Read the model definition and answer for the solid it produces. Units are mm, in the model's axes. A direction names the side the tool comes from. Round coordinates to 2 decimals unless told otherwise and drop trailing zeros. Order: outer loops, then holes, each group sorted by start corner. A loop starts at its lowest first (then second) coordinate and runs counter-clockwise, first axis right, second up. Notation, with made-up numbers: (-29.75, -12.75) - (-16.75, -12.75) arc R18 ccw to (-16.75, 3.25) - close; hole circle Ø1 at (-8.75, 39.5). An arc over 180 degrees is marked (long way). Put each result on its own line as item: value. Start each with the question number.
Q1. Which of the six approach directions +Z, -Z, +X, -X, +Y, -Y give full straight-line access (tool end or side, diameter ignored) to faces 5 (the face through (-58, 2, 10.445)), 6 (the face through (32.1, 2, -57)), 7 (the face through (-10.1, 2, 22)), 8 (the face through (-32.1, 2, 58))?
Q2. For a pull along Z with two mould halves and no side action, classify faces 1 (the face through (58, 2, -50.995)), 2 (the face through (52.3, 2, -57)), 3 (the face through (58, 2, 32.445)), 4 (the face through (0.112, 1.61, 39.757)) as pulls with the +Z half, pulls with the -Z half, needs draft (parallel to the pull), parting line crosses it, or undercut.
Q3. Each of these flat-tipped pins is pushed along its axis until it touches: pin 1 Ø1.5 at (y, z) = (1, -20.5) entering from +X; pin 2 Ø1 at (y, z) = (2, -19) entering from -X; pin 3 Ø1.6 at (x, y) = (-59.5, 2) entering from -Z (3 decimals). Where does it stop, or does it pass through?
Q4. Section B-B on z = 27.5 is taken. Give the vertices of the cut face in (x, y) (3 decimals).
Q5. Find the intervals of material crossed by line 1 along X through (y, z) = (1.75, -10); line 2 along Z through (x, y) = (-17, 1.7) (3 decimals); line 3 along Z through (x, y) = (-1, 3.05) (3 decimals), in increasing order. Write a range as from..to.
Q6. Section D-D on y = 1.1 is taken. State how many separate pieces and enclosed holes the cut face has, then the cut area to 3 significant figures.
Q7. Section C-C on x = -42.2 is taken. Give the vertices of the cut face in (y, z) (3 decimals), then the cut area to 3 significant figures.
Q8. Section A-A on x = -15 is taken. Give the vertices of the cut face in (y, z) (3 decimals), then the cut area to 3 significant figures.
from build123d import *

# Parameters (mm, degrees)
SKETCH2_W           = 126.6
SKETCH2_H           = 126.33
BOSS_EXTRUDE1_DEPTH = 3.175
SKETCH3_W           = 22
SKETCH3_H           = 22
CUT_EXTRUDE1_DEPTH  = 90.48065629
SKETCH4_R           = 2.55
CUT_EXTRUDE2_DEPTH  = 90.48065629


with BuildPart() as part:
    # Sketch2 → Boss-Extrude1 (new body)
    with BuildSketch(Plane(origin=(0, 0, 0), x_dir=(1, 0, 0), z_dir=(0, 1, 0))):
        Rectangle(SKETCH2_W, SKETCH2_H)
    extrude(amount=BOSS_EXTRUDE1_DEPTH)

    # Sketch3 → Cut-Extrude1 (cut, through all)
    with BuildSketch(Plane(origin=(0, 3.175, 0), x_dir=(1, 0, 0), z_dir=(0, 1, 0))):
        with Locations((63.3, -63.165)):
            Rectangle(SKETCH3_W, SKETCH3_H)
        with Locations((21.1, -63.165)):
            Rectangle(SKETCH3_W, SKETCH3_H)
        with Locations((-21.1, -63.165)):
            Rectangle(SKETCH3_W, SKETCH3_H)
        with Locations((-63.3, -63.165)):
            Rectangle(SKETCH3_W, SKETCH3_H)
        with Locations((21.1, -21.445)):
            Rectangle(SKETCH3_W, SKETCH3_H)
        with Locations((-21.1, -21.445)):
            Rectangle(SKETCH3_W, SKETCH3_H)
        with Locations((-63.3, -21.445)):
            Rectangle(SKETCH3_W, SKETCH3_H)
        with Locations((21.1, 20.275)):
            Rectangle(SKETCH3_W, SKETCH3_H)
        with Locations((-21.1, 20.275)):
            Rectangle(SKETCH3_W, SKETCH3_H)
        with Locations((-63.3, 20.275)):
            Rectangle(SKETCH3_W, SKETCH3_H)
        with Locations((21.1, 61.995)):
            Rectangle(SKETCH3_W, SKETCH3_H)
        with Locations((-21.1, 61.995)):
            Rectangle(SKETCH3_W, SKETCH3_H)
        with Locations((-63.3, 61.995)):
            Rectangle(SKETCH3_W, SKETCH3_H)
        with Locations((63.3, -21.445)):
            Rectangle(SKETCH3_W, SKETCH3_H)
        with Locations((63.3, 20.275)):
            Rectangle(SKETCH3_W, SKETCH3_H)
        with Locations((63.3, 61.995)):
            Rectangle(SKETCH3_W, SKETCH3_H)
    extrude(amount=-CUT_EXTRUDE1_DEPTH, mode=Mode.SUBTRACT)

    # Sketch4 → Cut-Extrude2 (cut, through all)
    with BuildSketch(Plane(origin=(0, 3.175, 0), x_dir=(1, 0, 0), z_dir=(0, 1, 0))):
        with Locations(Location((42.2, -42.305, 0), (0, 0, 270))):
            Circle(SKETCH4_R)
        with Locations(Location((0, -42.305, 0), (0, 0, 270))):
            Circle(SKETCH4_R)
        with Locations(Location((-42.2, -42.305, 0), (0, 0, 270))):
            Circle(SKETCH4_R)
        with Locations(Location((0, -0.585, 0), (0, 0, 270))):
            Circle(SKETCH4_R)
        with Locations(Location((-42.2, -0.585, 0), (0, 0, 270))):
            Circle(SKETCH4_R)
        with Locations(Location((0, 41.135, 0), (0, 0, 270))):
            Circle(SKETCH4_R)
        with Locations(Location((-42.2, 41.135, 0), (0, 0, 270))):
            Circle(SKETCH4_R)
        with Locations(Location((42.2, -0.585, 0), (0, 0, 270))):
            Circle(SKETCH4_R)
        with Locations(Location((42.2, 41.135, 0), (0, 0, 270))):
            Circle(SKETCH4_R)
    extrude(amount=-CUT_EXTRUDE2_DEPTH, mode=Mode.SUBTRACT)


solid = part.part
Findings:
1. face 5: -X, +Y, -Y
1. face 6: -Z, +Y, -Y
1. face 7: +Y, -Y
1. face 8: +Z, +Y, -Y
2. face 1: pulls with the -Z half
2. face 2: needs draft
2. face 3: undercut
2. face 4: undercut
3. pin 1: x = 52.3
3. pin 2: x = -52.3
3. pin 3: z = -50.995
4. outline: (-52.3, 0) - (-32.1, 0) - (-32.1, 3.175) - (-52.3, 3.175) - close; (-10.1, 0) - (10.1, 0) - (10.1, 3.175) - (-10.1, 3.175) - close; (32.1, 0) - (52.3, 0) - (52.3, 3.175) - (32.1, 3.175) - close
5. line 1: -52.3..-32.1, -10.1..10.1, 32.1..52.3
5. line 2: -50.995..-31.275, -9.275..10.445, 32.445..52.165
5. line 3: -63.165..-43.481, -38.789..-1.761, 2.931..39.959, 44.651..63.165
6. separate pieces: 1
6. enclosed holes: 13
6. area: 11,400 mm2
7. outline: (0, -63.165) - (3.175, -63.165) - (3.175, -43.685) - (0, -43.685) - close; (0, -38.585) - (3.175, -38.585) - (3.175, -1.965) - (0, -1.965) - close; (0, 3.135) - (3.175, 3.135) - (3.175, 39.755) - (0, 39.755) - close; (0, 44.855) - (3.175, 44.855) - (3.175, 63.165) - (0, 63.165) - close
7. area: 353 mm2
8. outline: (0, -50.995) - (3.175, -50.995) - (3.175, -31.275) - (0, -31.275) - close; (0, -9.275) - (3.175, -9.275) - (3.175, 10.445) - (0, 10.445) - close; (0, 32.445) - (3.175, 32.445) - (3.175, 52.165) - (0, 52.165) - close
8. area: 188 mm2
